Study the drawing (mm; zero at the part's minimum x, y, z) and answer. Coordinates: 2 decimals unless noted, no trailing zeros. Loops run counter-clockwise (first coordinate to the right, second up) from the corner with the lowest first, then second, coordinate; pieces in that order, holes last.
Q1. The mould has two halves that part along Y. Classify the marked faces 1, 2 and 3: pulls with the +Y half, pulls with the -Y half, needs draft (parallel to the pull), parting line crosses it, or undercut.
Q2. Section B-B (z = 4) is taken. Count the separate pieces of the cut face and the enclosed holes in it, then the cut area to 3 significant figures.
Q3. Section C-C (x = 31.75) is taken. Give the vertices of the cut face in (y, z), then the cut area to 3 significant figures.
Q4. Section D-D (y = 15.5) is taken. Give the vertices of the cut face in (x, z), then the cut area to 3 significant figures.
Q5. Section A-A (y = 25.4) is taken. Give the vertices of the cut face in (x, z), then the cut area to 3 significant figures.
Q6. Straight lines are drawn through the part: line 1 (Y direction, x = 31.75, z = 5); line 2 (X direction, y = 24.5, z = 1.5) (1 decimal); line 3 (Y direction, x = 27, z = 5) (1 decimal). For each, find the intervals that lie inside material, in ascending order.
Q7. A flat-ended cylindrical pin translates along its axis: P1, Ø5, axis at x = 57.94, y = 25.4, coming from the -Z side. Find the tip coordinate at first contact, or state that the pin passes through.
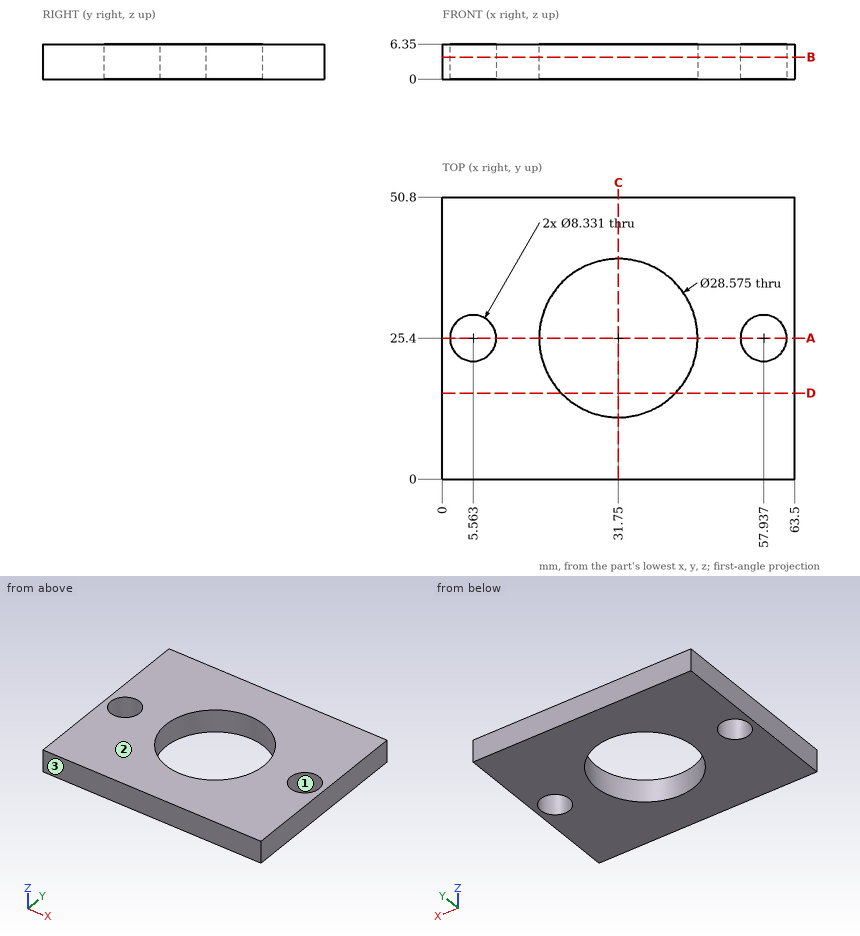
Numbers:
1. face 1: undercut
1. face 2: needs draft
1. face 3: pulls with the -Y half
2. separate pieces: 1
2. enclosed holes: 3
2. area: 2,480 mm2
3. outline: (0, 0) - (11.11, 0) - (11.11, 6.35) - (0, 6.35) - close; (39.69, 0) - (50.8, 0) - (50.8, 6.35) - (39.69, 6.35) - close
3. area: 141 mm2
4. outline: (0, 0) - (21.45, 0) - (21.45, 6.35) - (0, 6.35) - close; (42.05, 0) - (63.5, 0) - (63.5, 6.35) - (42.05, 6.35) - close
4. area: 272 mm2
5. outline: (0, 0) - (1.4, 0) - (1.4, 6.35) - (0, 6.35) - close; (9.73, 0) - (17.46, 0) - (17.46, 6.35) - (9.73, 6.35) - close; (46.04, 0) - (53.77, 0) - (53.77, 6.35) - (46.04, 6.35) - close; (62.1, 0) - (63.5, 0) - (63.5, 6.35) - (62.1, 6.35) - close
5. area: 116 mm2
6. line 1: y = 0 to 11.11, 39.69 to 50.8
6. line 2: x = 0 to 1.5, 9.6 to 17.5, 46 to 53.9, 62 to 63.5
6. line 3: y = 0 to 11.9, 38.9 to 50.8
7. P1: passes through
